from build123d import *

# Parameters (mm, degrees)
EXTRUDE_1_DEPTH     = 4
CUT_EXTRUDE_1_DEPTH = 10
FILLET_1_R          = 1


with BuildPart() as part:
    # 草图1 → 凸台-拉伸1 (new body)
    with BuildSketch(Plane.XY):
        Polygon((72.534285714, 6.73), (76.534285714, 6.73), (76.534285714, 16.23), (81.534285714, 16.23), (81.534285714, 24.23), (76.534285714, 24.23), (76.534285714, 33.73), (72.534285714, 33.73), (72.534285714, 32.38), (69.934285714, 32.38), (69.934285714, 33.73), (67.934285714, 33.73), (67.934285714, 36.73), (69.934285714, 36.73), (69.934285714, 38.08), (72.534285714, 38.08), (72.534285714, 36.73), (76.534285714, 36.73), (76.534285714, 46.23), (54.534285714, 46.23), (-91.465714286, 46.23), (-91.465714286, 36.73), (-87.465714286, 36.73), (-87.465714286, 38.08), (-84.865714286, 38.08), (-84.865714286, 36.73), (-82.865714286, 36.73), (-82.865714286, 33.73), (-84.865714286, 33.73), (-84.865714286, 32.38), (-87.465714286, 32.38), (-87.465714286, 33.73), (-91.465714286, 33.73), (-91.465714286, 24.23), (-96.465714286, 24.23), (-96.465714286, 16.23), (-91.465714286, 16.23), (-91.465714286, 6.73), (-87.465714286, 6.73), (-87.465714286, 8.08), (-84.865714286, 8.08), (-84.865714286, 6.73), (-82.865714286, 6.73), (-82.865714286, 3.73), (-84.865714286, 3.73), (-84.865714286, 2.38), (-87.465714286, 2.38), (-87.465714286, 3.73), (-91.465714286, 3.73), (-91.465714286, -5.77), (-96.465714286, -5.77), (-96.465714286, -13.77), (-91.465714286, -13.77), (-91.465714286, -23.27), (-87.465714286, -23.27), (-87.465714286, -21.92), (-84.865714286, -21.92), (-84.865714286, -23.27), (-82.865714286, -23.27), (-82.865714286, -26.27), (-84.865714286, -26.27), (-84.865714286, -27.62), (-87.465714286, -27.62), (-87.465714286, -26.27), (-91.465714286, -26.27), (-91.465714286, -35.77), (54.534285714, -35.77), (76.534285714, -35.77), (76.534285714, -26.27), (72.534285714, -26.27), (72.534285714, -27.62), (69.934285714, -27.62), (69.934285714, -26.27), (67.934285714, -26.27), (67.934285714, -23.27), (69.934285714, -23.27), (69.934285714, -21.92), (72.534285714, -21.92), (72.534285714, -23.27), (76.534285714, -23.27), (76.534285714, -13.77), (81.534285714, -13.77), (81.534285714, -5.77), (76.534285714, -5.77), (76.534285714, 3.73), (72.534285714, 3.73), (72.534285714, 2.38), (69.934285714, 2.38), (69.934285714, 3.73), (67.934285714, 3.73), (67.934285714, 6.73), (69.934285714, 6.73), (69.934285714, 8.08), (72.534285714, 8.08), align=None)
    extrude(amount=EXTRUDE_1_DEPTH)

    # 草图3 → 切除-拉伸1 (cut)
    with BuildSketch(Plane.XY.offset(4)):
        with BuildLine():
            Line((28.802924928, -16.42457109), (-74.094745974, 26.563182669))
            ThreePointArc((-74.094745974, 26.563182669), (-75.974331302, 26.382376332), (-76.865714286, 24.717753759))
            Line((-76.865714286, 24.717753759), (-76.865714286, -18.27))
            ThreePointArc((-76.865714286, -18.27), (-76.279927848, -19.684213562), (-74.865714286, -20.27))
            Line((-74.865714286, -20.27), (28.031956617, -20.27))
            ThreePointArc((28.031956617, -20.27), (29.992933136, -18.6631553), (28.802924928, -16.42457109))
        make_face()
        with BuildLine():
            Line((-42.963385188, 30.73), (59.934285714, 30.73))
            ThreePointArc((59.934285714, 30.73), (61.348499277, 30.144213562), (61.934285714, 28.73))
            Line((61.934285714, 28.73), (61.934285714, -14.257753759))
            ThreePointArc((61.934285714, -14.257753759), (61.042902731, -15.922376332), (59.163317403, -16.103182669))
            Line((59.163317403, -16.103182669), (-43.7343535, 26.88457109))
            ThreePointArc((-43.7343535, 26.88457109), (-44.924361708, 29.1231553), (-42.963385188, 30.73))
        make_face()
    extrude(amount=-CUT_EXTRUDE_1_DEPTH, mode=Mode.SUBTRACT)

    # 圆角1
    fillet_1_edges = [part.edges().sort_by_distance(p)[0] for p in [
        (-96.465714286, -13.77, 2),
        (-96.465714286, -5.77, 2),
        (-96.465714286, 16.23, 2),
        (-96.465714286, 24.23, 2),
        (81.534285714, 24.23, 2),
        (81.534285714, 16.23, 2),
        (81.534285714, -5.77, 2),
        (81.534285714, -13.77, 2),
    ]]
    fillet(fillet_1_edges, radius=FILLET_1_R)


solid = part.part
The listing builds one solid part. Answer for the finished solid, in the listing's coordinates (mm). A direction names the side the tool comes from. Coordinates: 2 decimals unless noted, no trailing zeros. Order: outer loops, then holes, each group sorted by start corner. A loop starts at its lowest first (then second) coordinate and runs counter-clockwise, first axis right, second up. Notation, with made-up numbers: M 87,76.5 L 109,76.5 A31 cw 109,110.5 Z; hole C -38.5,83 d3. An arc over 180 degrees is marked long. Use CSV: the item, a comma, the result in double quotes.
Q1. Section D-D (z = 1.6) is taken. Give the number of separate pieces and of enclosed holes in the cut face, then the cut area to 3 significant figures.
Here are the results:
separate pieces,"1"
enclosed holes,"2"
area,"8,260 mm2"
Q2. A tool of negligible diameter and unlimited length cuts with its end or side. For faces 5 (the flat face through (-91.466, 42, 2)), 6 (the flat face through (-24, -20.27, 2)), 7 (the flat face through (-82.866, -25, 2)), 8 (the flat face through (75, -23.27, 2)), from which of +Z, -Z, +X, -X, +Y, -Y can it reach the whole face along a straight path? Write none if from no direction.
Here are the results:
face 5,"+Z, -Z, -X, +Y"
face 6,"+Z, -Z"
face 7,"+Z, -Z, -X"
face 8,"+Z, -Z, +X"
Q3. Given pin 1 Ø1.2 at (y, z) = (29, 2.5) entering from +X; pin 2 Ø1.1 at (y, z) = (-23, 2) entering from -X; pin 3 Ø1.2 at (x, z) = (-92.5, 3) entering from -Y, each flat-ended and moving along its own axis, determine where each tip first touches the part or whether it passes through.
Here are the results:
pin 1,"x = 76.53"
pin 2,"x = -91.47"
pin 3,"y = -13.77"
Q4. Straight lines are drawn through the part: L1, parallel to Y at x = 69.5, z = 2.3; L2, parallel to Y at x = -85.5, z = 1.65; L3, parallel to Y at x = -68.5, z = 1.75. For each, find the intervals that lie inside material, in ascending order.
Here are the results:
L1,"-35.77 to -26.27, -23.27 to 3.73, 6.73 to 33.73, 36.73 to 46.23"
L2,"-35.77 to -27.62, -21.92 to 2.38, 8.08 to 32.38, 38.08 to 46.23"
L3,"-35.77 to -20.27, 24.23 to 46.23"
Q5. Section B-B (x = -3.5) is taken. Determine the outline of the cut face in (y, z), then the cut area to 3 significant figures.
Here are the results:
outline,"M -35.77,0 L -20.27,0 L -20.27,4 L -35.77,4 Z; M -2.93,0 L 10.08,0 L 10.08,4 L -2.93,4 Z; M 30.73,0 L 46.23,0 L 46.23,4 L 30.73,4 Z"
area,"176 mm2"
Q6. Section A-A (x = 43) is taken. Determine the outline of the cut face in (y, z).
Here are the results:
outline,"M -35.77,0 L -9.35,0 L -9.35,4 L -35.77,4 Z; M 30.73,0 L 46.23,0 L 46.23,4 L 30.73,4 Z"
Q7. Section C-C (y = -1) is taken. Determine the outline of the cut face in (x, z), then the cut area to 3 significant figures.
Here are the results:
outline,"M -91.47,0 L -76.87,0 L -76.87,4 L -91.47,4 Z; M -8.12,0 L 23.01,0 L 23.01,4 L -8.12,4 Z; M 61.93,0 L 76.53,0 L 76.53,4 L 61.93,4 Z"
area,"241 mm2"
Q8. Determine the mould class of faces 1 (the flat face through (75, 6.73, 2)), 2 (the flat face through (-96.466, -10, 2)), 3 (the flat face through (79, 24.23, 2)), 4 (the flat face through (-89, 36.73, 2)) for opening direction Y: pulls with the +Y half, pulls with the -Y half, needs draft (parallel to the pull), parting line crosses it, or undercut.
Here are the results:
face 1,"undercut"
face 2,"needs draft"
face 3,"pulls with the +Y half"
face 4,"undercut"
